CAD build for the part. Positions are in the model's coordinates, mm. A direction names the side the tool comes from. Give positions to 0.01 mm unless a question says otherwise; leave off trailing zeros. Loops run counter-clockwise (first coordinate to the right, second up) from the corner with the lowest first, then second, coordinate; pieces in that order, holes last. Notation, with made-up numbers: (-34, 51.5) -> (-25, 51.5) arc R21 cw to (-25, 76.5) -> close; hole circle Ø11 at (10, 30). An arc over 180 degrees is marked (long way). Use one line per item in the form item = value.
```python
from build123d import *

# Parameters (mm, degrees)
SKETCH2_W           = 30
SKETCH2_H           = 4.3
BOSS_EXTRUDE1_DEPTH = 4.3


with BuildPart() as part:
    # Sketch2 → Boss-Extrude1 (new body)
    with BuildSketch(Plane.XY):
        Polygon((100, 0), (100, 17.35), (104.7, 17.35), (104.7, 32.65), (100, 32.65), (100, 47.35), (104.7, 47.35), (104.7, 62.65), (100, 62.65), (100, 77.35), (104.7, 77.35), (104.7, 92.65), (100, 92.65), (100, 107.35), (104.7, 107.35), (104.7, 122.65), (100, 122.65), (100, 140), (86.275, 140), (86.275, 135.3), (71.275, 135.3), (71.275, 140), (57.5, 140), (57.5, 135.3), (42.5, 135.3), (42.5, 140), (28.725, 140), (28.725, 135.3), (13.725, 135.3), (13.725, 140), (0, 140), (0, 82), (4.7, 82), (4.7, 62), (0, 62), (0, 0), (13.575, 0), (13.575, -4.3), (28.875, -4.3), (28.875, 0), (42.35, 0), (42.35, -4.3), (57.65, -4.3), (57.65, 0), (71.125, 0), (71.125, -4.3), (86.425, -4.3), (86.425, 0), align=None)
        with Locations((50, 49.85)):
            Rectangle(SKETCH2_W, SKETCH2_H, mode=Mode.SUBTRACT)
        with Locations((50, 94.15)):
            Rectangle(SKETCH2_W, SKETCH2_H, mode=Mode.SUBTRACT)
    extrude(amount=BOSS_EXTRUDE1_DEPTH)


solid = part.part
```
1. Cut at B-B, the plane z = 3.35. State how many separate pieces and enclosed holes the cut face has, then the cut area to 3 significant figures.
Result sheet:
separate_pieces = 1
enclosed_holes = 2
area = 13,900 mm^2
2. Cut at A-A, the plane x = 52. Write the cut outline in (y, z).
Result sheet:
outline = (-4.3, 0) -> (47.7, 0) -> (47.7, 4.3) -> (-4.3, 4.3) -> close; (52, 0) -> (92, 0) -> (92, 4.3) -> (52, 4.3) -> close; (96.3, 0) -> (135.3, 0) -> (135.3, 4.3) -> (96.3, 4.3) -> close
3. Cut at C-C, the plane x = 94. Write the cut outline in (y, z).
Result sheet:
outline = (0, 0) -> (140, 0) -> (140, 4.3) -> (0, 4.3) -> close
4. Cut at D-D, the plane x = 26.5. Write the cut outline in (y, z).
Result sheet:
outline = (-4.3, 0) -> (135.3, 0) -> (135.3, 4.3) -> (-4.3, 4.3) -> close
5. Tool access for faces 1 (the flat face through (102, 32.65, 2)), 2 (the flat face through (64, 0, 2)), 3 (the flat face through (57.5, 138, 2)): list every direction of +Z, -Z, +X, -X, +Y, -Y with a clear straight run to the whole face (end or side of a thin tool).
Result sheet:
face_1 = +Z, -Z, +X
face_2 = +Z, -Z, -Y
face_3 = +Z, -Z, +Y
6. Drill centre lines: line 1 (Y direction, x = 38.5, z = 0.4); line 2 (Y direction, x = 46, z = 1.35); line 3 (Y direction, x = 94, z = 0.9). Where is each one in solid material? Low to high.
Result sheet:
line_1 = 0 to 47.7, 52 to 92, 96.3 to 140
line_2 = -4.3 to 47.7, 52 to 92, 96.3 to 135.3
line_3 = 0 to 140
7. Drop flat-ended pins along their axis: P1, Ø1.3, axis at x = 102, z = 2, coming from the +Y side; P2, Ø2, axis at y = 36.5, z = 1.5, coming from the +X side; P3, Ø2, axis at x = 48.5, z = 1.5, coming from the +Y side. Give the stop position or say it passes through.
Result sheet:
P1 = 122.65
P2 = 100
P3 = 135.3
8. Mould opens along X. For faces 4 (the flat face through (4.7, 72, 2)), 5 (the flat face through (86.425, -2, 2)), 6 (the flat face through (35, 94, 2)), 7 (the flat face through (102, 17.35, 2)) say: pulls with the +X half, pulls with the -X half, needs draft (parallel to the pull), parting line crosses it, or undercut.
Result sheet:
face_4 = pulls with the -X half
face_5 = pulls with the +X half
face_6 = undercut
face_7 = needs draft
